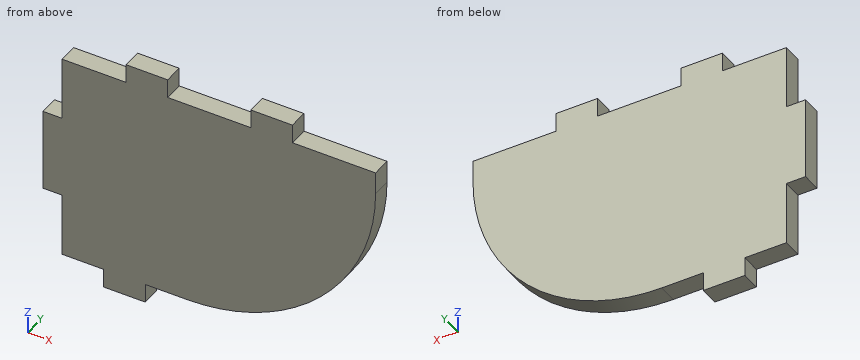
from build123d import *

# Parameters (mm, degrees)
SKETCH1_W          = 50.8
SKETCH1_H          = 38.1
EXTRUDE_2_DEPTH    = 2.921
FRONT_TABS_DEPTH   = 64.567147498
SIDE_TAB_DEPTH     = 64.567147498
CUT_EXTRUDE2_DEPTH = 64.567147498


with BuildPart() as part:
    # Sketch1 → extrude 2 (new body)
    with BuildSketch(Plane(origin=(0, 0, 0), x_dir=(1, 0, 0), z_dir=(0, 1, 0))):
        with Locations((25.4, 19.05)):
            Rectangle(SKETCH1_W, SKETCH1_H)
    extrude(amount=EXTRUDE_2_DEPTH)

    # Sketch2 → front tabs (cut, through all)
    with BuildSketch(Plane(origin=(0, 2.921, 0), x_dir=(1, 0, 0), z_dir=(0, 1, 0))):
        Polygon((0, -13.073373741), (50.8, -13.073373741), (50.8, 2.921), (38.1, 2.921), (38.1, -7.014658109), (31.75, -7.014658109), (31.75, 2.921), (19.05, 2.921), (19.05, -5.986156243), (12.7, -5.986156243), (12.7, 2.921), (0, 2.921), align=None)
    extrude(amount=-FRONT_TABS_DEPTH, mode=Mode.SUBTRACT)

    # Sketch3 → side tab (cut, through all)
    with BuildSketch(Plane(origin=(0, 2.921, 0), x_dir=(1, 0, 0), z_dir=(0, 1, 0))):
        Polygon((2.921, 25.4), (-4.31094219, 25.4), (-4.31094219, 12.7), (2.921, 12.7), (2.921, 0), (-6.847135587, 0), (-6.847135587, 38.1), (2.921, 38.1), align=None)
    extrude(amount=-SIDE_TAB_DEPTH, mode=Mode.SUBTRACT)

    # Sketch5 → Cut-Extrude2 (cut, through all)
    with BuildSketch(Plane(origin=(0, 2.921, 0), x_dir=(1, 0, 0), z_dir=(0, 1, 0))):
        with BuildLine():
            Line((-6.071846443, 35.179), (9.271, 35.179))
            Line((9.271, 35.179), (9.271, 42.517295463))
            Line((9.271, 42.517295463), (15.621, 42.517295463))
            Line((15.621, 42.517295463), (15.621, 35.179))
            Line((15.621, 35.179), (21.971, 35.179))
            ThreePointArc((21.971, 35.179), (42.356181395, 26.735181395), (50.8, 6.35))
            Line((50.8, 6.35), (50.8, 2.921))
            Line((50.8, 2.921), (62.623975616, 47.008361676))
            Line((62.623975616, 47.008361676), (-4.438145021, 50.333756088))
            Line((-4.438145021, 50.333756088), (-6.071846443, 35.179))
        make_face()
    extrude(amount=-CUT_EXTRUDE2_DEPTH, mode=Mode.SUBTRACT)


solid = part.part
Can you work these out from the model? Positions are in its coordinate system, mm. Give positions to 0.01 mm unless a question says otherwise; leave off trailing zeros. Loops run counter-clockwise (first coordinate to the right, second up) from the corner with the lowest first, then second, coordinate; pieces in that order, holes last. Notation, with made-up numbers: (37, -9) -> (68, -9) arc R29 ccw to (68, 25) -> close; hole circle Ø7 at (86.25, 21). An arc over 180 degrees is marked (long way). Write item = value, one per line.
1) Suppose I cut it at A-A on y = 1.4. Write out the boundary of the cut face in (x, z), then the cut area to 3 significant figures.
Check result:
outline = (0, -25.4) -> (2.92, -25.4) -> (2.92, -35.18) -> (9.27, -35.18) -> (9.27, -38.1) -> (15.62, -38.1) -> (15.62, -35.18) -> (21.97, -35.18) arc R28.83 ccw to (50.8, -6.35) -> (50.8, -2.92) -> (38.1, -2.92) -> (38.1, 0) -> (31.75, 0) -> (31.75, -2.92) -> (19.05, -2.92) -> (19.05, 0) -> (12.7, 0) -> (12.7, -2.92) -> (2.92, -2.92) -> (2.92, -12.7) -> (0, -12.7) -> close
area = 1,460 mm2
2) Suppose I cut it at C-C on z = -22.5. Write out the boundary of the cut face in (x, y).
Check result:
outline = (0, 0) -> (45.85, 0) -> (45.85, 2.92) -> (0, 2.92) -> close
3) Will these pins go through, and if not, where does the flat tip stop? pin 1 (1.5 mm diameter, centred on y = 2, z = -2, fed in from -X); pin 2 (10 mm diameter, centred on x = 6, z = -31.5, fed in from -Y); pin 3 (1.5 mm diameter, centred on x = 5.5, y = 2, fed in from -Z); pin 4 (1.5 mm diameter, centred on x = 25.5, y = 1, fed in from +Z).
Check result:
pin_1 = 12.7
pin_2 = 0
pin_3 = -35.18
pin_4 = -2.92
4) Suppose I cut it at B-B on x = 11. Write out the boundary of the cut face in (y, z).
Check result:
outline = (0, -38.1) -> (2.92, -38.1) -> (2.92, -2.92) -> (0, -2.92) -> close
5) I need wall thicknesses on L1, parallel to X at y = 0.1, z = -1.5; L2, parallel to X at y = 0.65, z = -3; L3, parallel to Z at x = 10, y = 1.15. Which ranges of each line are inside material? Lowest first, please. Write a range as from..to.
Check result:
L1 = 12.7..19.05, 31.75..38.1
L2 = 2.92..50.8
L3 = -38.1..-2.92
